from build123d import *

# Parameters (mm, degrees)
SKETCH1_W                = 332
SKETCH1_H                = 16
BOSS_EXTRUDE1_DEPTH      = 8
SHELL1_T                 = -1
SKETCH2_W                = 4
SKETCH2_H                = 16
BOSS_EXTRUDE2_DEPTH      = 48
BOSS_EXTRUDE2_DEPTH_BACK = 15
BOSS_EXTRUDE3_START      = -16
BOSS_EXTRUDE3_DEPTH      = 18
CUT_EXTRUDE1_DEPTH       = 40
FILLET1_R                = 5
FILLET2_R                = 2
FILLET1_OF_MIRROR1_R     = 5
FILLET2_OF_MIRROR1_R     = 2
SKETCH1_3_R              = 3.175
CUT_EXTRUDE2_DEPTH       = 48.5
CUT_EXTRUDE2_DEPTH_BACK  = 48.5


with BuildPart() as part:
    # Sketch1 → Boss-Extrude1 (new body, symmetric)
    with BuildSketch(Plane.XY):
        with Locations((-206, 0)):
            Rectangle(SKETCH1_W, SKETCH1_H)
    extrude(amount=BOSS_EXTRUDE1_DEPTH, both=True)

    # Shell1
    shell1_openings = [part.faces().sort_by_distance(p)[0] for p in [
        (-40, 0, 0),
        (-372, 0, 0),
    ]]
    offset(amount=SHELL1_T, openings=shell1_openings, kind=Kind.INTERSECTION)

    # Sketch2 → Boss-Extrude2 (add, two sides)
    with BuildSketch(Plane(origin=(-40, 0, 0), x_dir=(0, 0, -1), z_dir=(1, 0, 0))) as boss_extrude2_sk:
        with Locations((-10, 0)):
            Rectangle(SKETCH2_W, SKETCH2_H)
        with Locations((10, 0)):
            Rectangle(SKETCH2_W, SKETCH2_H)
    extrude(amount=BOSS_EXTRUDE2_DEPTH)
    extrude(boss_extrude2_sk.sketch, amount=-BOSS_EXTRUDE2_DEPTH_BACK)

    # Sketch3 → Boss-Extrude3 (add)
    with BuildSketch(Plane(origin=(0, 8, 0), x_dir=(1, 0, 0), z_dir=(0, 1, 0)).offset(BOSS_EXTRUDE3_START)):
        Polygon((-336, -14), (-336, -8), (-372, -8), (-413, -41.5), (-522, -41.5), (-522, -47.5), (-413, -47.5), (-372, -14), align=None)
    boss_extrude3 = extrude(amount=BOSS_EXTRUDE3_DEPTH)

    # Sketch4 → Cut-Extrude1 (cut)
    with BuildSketch(Plane.XY.offset(47.5)):
        with BuildLine():
            Line((-510, 10), (-518.823529412, 5.294117647))
            ThreePointArc((-518.823529412, 5.294117647), (-521.99760764, -0.169418391), (-518.520172623, -5.445064733))
            Line((-518.520172623, -5.445064733), (-513, -8))
            Line((-513, -8), (-540.277730866, -26.369352849))
            Line((-540.277730866, -26.369352849), (-542.314823198, 28.070412495))
            Line((-542.314823198, 28.070412495), (-510, 10))
        make_face()
    cut_extrude1 = extrude(amount=-CUT_EXTRUDE1_DEPTH, mode=Mode.SUBTRACT)

    # Fillet1
    fillet1_edges = [part.edges().sort_by_distance(p)[0] for p in [
        (-413, 1, 41.5),
        (-413, 1, 47.5),
        (-372, 1, 14),
        (-372, 9, 8),
    ]]
    fillet(fillet1_edges, radius=FILLET1_R)

    # Fillet2
    fillet2_edges = [part.edges().sort_by_distance(p)[0] for p in [
        (-462.391472159, 10, 47.5),
        (-392.5, 10, 30.75),
        (-413.103576447, 10, 47.209535386),
        (-353.108527841, -8, 14),
        (-392.5, -8, 30.75),
        (-413.103576447, -8, 47.209535386),
        (-371.896423553, -8, 14.290464614),
        (-371.896423553, 10, 14.290464614),
        (-353.108527841, 10, 14),
        (-336, 1, 14),
        (-463.891472159, -8, 47.5),
        (-521.99760764, -0.169418391, 47.5),
        (-514.411764706, 7.647058824, 47.5),
        (-515.760086311, -6.722532367, 47.5),
    ]]
    fillet(fillet2_edges, radius=FILLET2_R)

    # Mirror1: Boss-Extrude3, Cut-Extrude1 across plane
    add(boss_extrude3.mirror(Plane.XY))
    add(cut_extrude1.mirror(Plane.XY), mode=Mode.SUBTRACT)

    # Fillet1 of Mirror1
    fillet1_of_mirror1_edges = [part.edges().sort_by_distance(p)[0] for p in [
        (-413, 1, -41.5),
        (-413, 1, -47.5),
        (-372, 1, -14),
        (-372, 9, -8),
    ]]
    fillet(fillet1_of_mirror1_edges, radius=FILLET1_OF_MIRROR1_R)

    # Fillet2 of Mirror1
    fillet2_of_mirror1_edges = [part.edges().sort_by_distance(p)[0] for p in [
        (-462.391472159, 10, -47.5),
        (-392.5, 10, -30.75),
        (-413.103576447, 10, -47.209535386),
        (-353.108527841, -8, -14),
        (-392.5, -8, -30.75),
        (-413.103576447, -8, -47.209535386),
        (-371.896423553, -8, -14.290464614),
        (-371.896423553, 10, -14.290464614),
        (-353.108527841, 10, -14),
        (-336, 1, -14),
        (-463.891472159, -8, -47.5),
        (-521.99760764, -0.169418391, -47.5),
        (-514.411764706, 7.647058824, -47.5),
        (-515.760086311, -6.722532367, -47.5),
    ]]
    fillet(fillet2_of_mirror1_edges, radius=FILLET2_OF_MIRROR1_R)

    # Sketch1<3> → Cut-Extrude2 (cut, two sides)
    with BuildSketch(Plane.XY) as cut_extrude2_sk:
        with Locations((-516, 0)):
            Circle(SKETCH1_3_R)
        Circle(SKETCH1_3_R)
    extrude(amount=CUT_EXTRUDE2_DEPTH, mode=Mode.SUBTRACT)
    extrude(cut_extrude2_sk.sketch, amount=-CUT_EXTRUDE2_DEPTH_BACK, mode=Mode.SUBTRACT)


solid = part.part
Verification items for the finished model (mm, model axes). A direction names the side the tool comes from. Give positions to 0.01 mm unless a question says otherwise; leave off trailing zeros. Write each loop counter-clockwise with the first axis right and the second up, starting at its lowest first coordinate (ties: lowest second). Pieces come first, ordered by that corner, then holes. Notation, with made-up numbers: M 13,17.25 L 19,17.25 A26 ccw 19,53.25 Z; hole C 89.25,7.25 d11. An arc over 180 degrees is marked long. Use CSV: the item, a comma, the result in double quotes.
1) Material ranges on line 1 along X through (y, z) = (0, 10.2) (3 decimals); line 2 along Z through (x, y) = (-327, 0); line 3 along Z through (x, y) = (-464, 3), recorded low to high.
Final values:
line 1,"-374.693 to -336, -55 to -3.175, 3.175 to 8"
line 2,"-8 to -7, 7 to 8"
line 3,"-47.5 to -41.5, 41.5 to 47.5"
2) Cross-section at C-C (y = 0). State how many separate pieces and enclosed holes the cut face has, plus the area to 3 significant figures.
Final values:
separate pieces,"6"
enclosed holes,"0"
area,"3,270 mm²"
3) Go/stop test with flat-tipped pins: pin 1 Ø7 at (x, z) = (-164, 2.5) entering from +Y; pin 2 Ø8 at (x, y) = (-7, 2) entering from -Z; pin 3 Ø4 at (y, z) = (0.5, 31.5) entering from +X. Record where each tip stops, or that it passes through.
Final values:
pin 1,"y = 8"
pin 2,"z = -12"
pin 3,"x = -390.97"
4) Cross-section at A-A (x = -317.5). Enter the section's corners in (y, z), plus the area to 3 significant figures.
Final values:
outline,"M -8,-8 L 8,-8 L 8,8 L -8,8 Z; hole M -7,-7 L 7,-7 L 7,7 L -7,7 Z"
area,"60.0 mm²"
5) Release check for a two-part mould opening along Z. For faces 6 (the face through (-468, 1, 41.5)), 7 (the face through (-423, 10, -42)), 8 (the face through (-23, 0, 12)), 9 (the face through (-468, 1, -41.5)) record: released by +Z, released by -Z, zero draft, split by the parting line, or undercut.
Final values:
face 6,"undercut"
face 7,"zero draft"
face 8,"released by +Z"
face 9,"undercut"
6) Cross-section at B-B (z = -1.5). Enter the section's corners in (x, y).
Final values:
outline,"M -372,-8 L -40,-8 L -40,-7 L -372,-7 Z; M -372,7 L -40,7 L -40,8 L -372,8 Z"
7) Access from +Z, -Z, +X, -X, +Y, -Y to the whole of each face (thin tool, end or side, straight path). Record for faces 1 (the face through (-391.53, 0.87, 23.96)), 2 (the face through (-354, 1, -14)), 3 (the face through (-208, 0, 7)), 4 (the face through (-16, 0, 8)), 5 (the face through (-234, -8, 0)).
Final values:
face 1,"-X, +Y, -Y"
face 2,"-Z, +X, +Y, -Y"
face 3,"+X, -X"
face 4,"+X, +Y, -Y"
face 5,"+Z, -Z, +X, -X, -Y"
